from build123d import *

# Parameters (mm, degrees)
F0_W     = 101.395164
F0_H     = 34.843063
F1_DEPTH = 25.4
F2_R     = 6.038851
F2_R_2   = 5.643182
F3_DEPTH = 46.99
F4_W     = 62.337181
F4_H     = 34.332353
F5_DEPTH = 30.48


with BuildPart() as f1:
    # F0 (on Front) → F1 (new body)
    with BuildSketch(Plane.XZ):
        with BuildLine():
            Line((-50.236695, -23.689596), (-50.236695, 11.153467))
            ThreePointArc((-50.236695, 11.153467), (-67.658226, -6.268064), (-50.236695, -23.689596))
        make_face()
        with Locations((0.460887, -6.268064)):
            Rectangle(F0_W, F0_H)
        with BuildLine():
            ThreePointArc((51.158469, -23.689596), (68.580001, -6.268064), (51.158469, 11.153467))
            Line((51.158469, 11.153467), (51.158469, -23.689596))
        make_face()
    extrude(amount=F1_DEPTH)

    # F2 (on Front) → F3 (cut)
    with BuildSketch(Plane.XZ):
        with Locations((-53.002015, -5.622823)):
            Circle(F2_R)
        with Locations((54.292504, -5.622823)):
            Circle(F2_R_2)
    extrude(amount=F3_DEPTH, mode=Mode.SUBTRACT)

    # F4 (on Front) → F5 (join)
    with BuildSketch(Plane.XZ):
        with Locations((-1.877168, -6.187636)):
            Rectangle(F4_W, F4_H)
    extrude(amount=-F5_DEPTH)


solid = f1.part
Input: part model. Units: mm. Frame: model coordinates. A direction names the side the tool comes from. Coordinates: 2 decimals unless noted, no trailing zeros. Order: outer loops, then holes, each group sorted by start corner. A loop starts at its lowest first (then second) coordinate and runs counter-clockwise, first axis right, second up. Notation, with made-up numbers: M -10.75,51 L 46.25,51 A14 cw 46.25,60 Z; hole C 4,-24.75 d6. An arc over 180 degrees is marked long. Write item = value, one per line. Start each with the question number.
(1) Section A-A on x = -52. Output: boundary loops of the cut face in (y, z).
(2) Section B-B on y = -20. Output: boundary loops of the cut face in (x, z).
(3) Line query: line 1 along X through (y, z) = (-6.5, -1.5); line 2 along X through (y, z) = (-6.5, -6.5); line 3 along Y through (x, z) = (50, -21). Output: solid intervals per line, ascending. Write a range as [from, to].
(4) Reachability of faces 1 (the flat face through (-2, 15, 10.979)), 2 (the flat face through (-33.046, 15, -6)), 3 (the cylindrical face through (68.576, -12.522, -6.651)), 4 (the flat face through (-2, 15, -23.354)), 5 (the flat face through (0, -25.4, -6)) from +Z, -Z, +X, -X, +Y, -Y: full face, straight path, thin tool, end or side. Return the list, or none.
(5) First-contact query: P1, Ø12, axis at x = 3.5, y = 9, coming from the +Z side; P2, Ø9, axis at x = 54.29, z = -5.62, coming from the +Y side; P3, Ø9, axis at y = 17, z = -1.5, coming from the +X side; P4, Ø9, axis at y = 14, z = -7.5, coming from the -X side. Flat tips, straight axial feed; report the tip coordinate or a pass-through.
(6) Pull-direction query (Z, two-part tool) for faces 6 (the flat face through (29.291, 15, -6)), 7 (the cylindrical face through (-47.24, -12.52, -3.81)), 8 (the flat face through (0, -13, -23.69)); classes: released by +Z, released by -Z, zero draft, split by the parting line, or undercut.
(7) Section C-C on z = -19. Output: boundary loops of the cut face in (x, y), and give its area (3 significant figures).
(8) Section D-D on y = 7. Output: boundary loops of the cut face in (x, z), and give its area (3 significant figures).
Result set:
q1.outline = M -25.4,-23.6 L 0,-23.6 L 0,-11.58 L -25.4,-11.58 Z; M -25.4,0.33 L 0,0.33 L 0,11.06 L -25.4,11.06 Z
q2.outline = M -50.24,-23.69 L 51.16,-23.69 A17.42 ccw 51.16,11.15 L -50.24,11.15 A17.42 ccw Z; hole C -53,-5.62 d12.08; hole C 54.29,-5.62 d11.29
q3.line_1 = [-66.99, -57.41], [-48.59, 50.44], [58.15, 67.91]
q3.line_2 = [-67.66, -58.98], [-47.03, 48.72], [59.87, 68.58]
q3.line_3 = [-25.4, 0]
q4.face_1 = +Z, +X, -X, +Y
q4.face_2 = +Z, -Z, -X, +Y
q4.face_3 = +X, +Y, -Y
q4.face_4 = -Z, +X, -X, +Y
q4.face_5 = +Z, -Z, +X, -X, -Y
q5.P1 = 10.98
q5.P2 = through
q5.P3 = 29.29
q5.P4 = -33.05
q6.face_6 = zero draft
q6.face_7 = undercut
q6.face_8 = released by -Z
q7.outline = M -62.13,-25.4 L 63.05,-25.4 L 63.05,0 L 29.29,0 L 29.29,30.48 L -33.05,30.48 L -33.05,0 L -62.13,0 Z
q7.area = 5,080 mm²
q8.outline = M -33.05,-23.35 L 29.29,-23.35 L 29.29,10.98 L -33.05,10.98 Z
q8.area = 2,140 mm²
